Read the model definition and answer for the solid it produces. Units are mm, in the model's axes. Face numbers are marked on the shaded views. A direction names the side the tool comes from. Coordinates: 2 decimals unless noted, no trailing zeros. Loops run counter-clockwise (first coordinate to the right, second up) from the corner with the lowest first, then second, coordinate; pieces in that order, holes last.
from build123d import *

# Parameters (mm, degrees)
SKETCH4_R           = 31.5
SKETCH4_R_2         = 21.5
SKETCH4_R_3         = 2
BOSS_EXTRUDE1_DEPTH = 4
SKETCH5_W           = 97.16267939
SKETCH5_H           = 14.406328081
SKETCH5_H_2         = 19.608613221
CUT_EXTRUDE1_DEPTH  = 66


with BuildPart() as part:
    # Sketch1 → Revolve1 (revolve)
    with BuildSketch(Plane.XY):
        Polygon((-12, 2.5), (-12, -2.5), (-16, -2.5), (-16, -18.5), (-20, -18.5), (-20, -32.5), (-23, -32.5), (-23, 32.5), (-20, 32.5), (-20, 18.5), (-16, 18.5), (-16, 2.5), align=None)
    revolve(axis=Axis((0, 75.096781517, 0), (0, -1, 0)))

    # Sketch4 → Boss-Extrude1 (add)
    with BuildSketch(Plane(origin=(0, 32.5, 0), x_dir=(1, 0, 0), z_dir=(0, 1, 0))):
        Circle(SKETCH4_R)
        Circle(SKETCH4_R_2, mode=Mode.SUBTRACT)
        with Locations((0, 27)):
            Circle(SKETCH4_R_3, mode=Mode.SUBTRACT)
        with Locations((19.091883092, 19.091883092)):
            Circle(SKETCH4_R_3, mode=Mode.SUBTRACT)
        with Locations((27, 0)):
            Circle(SKETCH4_R_3, mode=Mode.SUBTRACT)
        with Locations((19.091883092, -19.091883092)):
            Circle(SKETCH4_R_3, mode=Mode.SUBTRACT)
        with Locations((0, -27)):
            Circle(SKETCH4_R_3, mode=Mode.SUBTRACT)
        with Locations((-19.091883092, -19.091883092)):
            Circle(SKETCH4_R_3, mode=Mode.SUBTRACT)
        with Locations((-27, 0)):
            Circle(SKETCH4_R_3, mode=Mode.SUBTRACT)
        with Locations((-19.091883092, 19.091883092)):
            Circle(SKETCH4_R_3, mode=Mode.SUBTRACT)
    boss_extrude1 = extrude(amount=-BOSS_EXTRUDE1_DEPTH)

    # Mirror1: Boss-Extrude1 across plane
    add(boss_extrude1.mirror(Plane.ZX))

    # Sketch5 → Cut-Extrude1 (cut, through all)
    with BuildSketch(Plane(origin=(0, 32.5, 0), x_dir=(1, 0, 0), z_dir=(0, 1, 0))):
        with Locations((4.630564128, 32.20316404)):
            Rectangle(SKETCH5_W, SKETCH5_H)
        with Locations((4.630564128, -34.804306611)):
            Rectangle(SKETCH5_W, SKETCH5_H_2)
    extrude(amount=-CUT_EXTRUDE1_DEPTH, mode=Mode.SUBTRACT)


solid = part.part
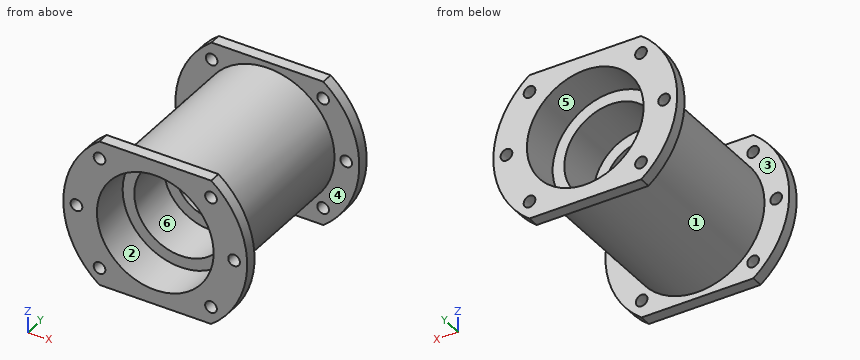
Item 1: Given pin 1 (3 mm diameter, centred on x = 27, z = 0, fed in from +Y); pin 2 (12 mm diameter, centred on x = -5.5, z = -5.5, fed in from -Y); pin 3 (1 mm diameter, centred on y = -24, z = -4.5, fed in from -X); pin 4 (5 mm diameter, centred on x = 17.5, z = 3, fed in from -Y), each flat-ended and moving along its own axis, determine where each tip first touches the part or whether it passes through.
Numbers:
pin 1: passes through
pin 2: stops at y = -2.5
pin 3: stops at x = -22.65
pin 4: stops at y = -32.5
Item 2: A cutting plane is placed at C-C on y = 0.5. Determine the outline of the cut face in (x, z).
Numbers:
outline: circle Ø46 at (0, 0); hole circle Ø24 at (0, 0)
Item 3: Which of the six approach directions +Z, -Z, +X, -X, +Y, -Y give full straight-line access (tool end or side, diameter ignored) to the marked faces 4, 5 and 6?
Numbers:
face 4: none
face 5: +Y
face 6: -Y
Item 4: A cutting plane is placed at B-B on x = -27. Determine the outline of the cut face in (y, z), then the cut area to 3 significant figures.
Numbers:
outline: (-32.5, -16.22) - (-28.5, -16.22) - (-28.5, -2) - (-32.5, -2) - close; (-32.5, 2) - (-28.5, 2) - (-28.5, 16.22) - (-32.5, 16.22) - close; (28.5, -16.22) - (32.5, -16.22) - (32.5, -2) - (28.5, -2) - close; (28.5, 2) - (32.5, 2) - (32.5, 16.22) - (28.5, 16.22) - close
area: 228 mm2
Item 5: A cutting plane is placed at D-D on z = 0. Give the number of separate pieces and of enclosed holes in the cut face, then the cut area to 3 significant figures.
Numbers:
separate pieces: 6
enclosed holes: 0
area: 798 mm2
Item 6: Find the intervals of material crossed by line 1 along Y through (x, z) = (-20.5, -13); line 2 along Z through (x, y) = (0, 8); line 3 along Z through (x, y) = (0, 28), in increasing order.
Numbers:
line 1: y = -32.5 to -28.5, 28.5 to 32.5
line 2: z = -23 to -16, 16 to 23
line 3: z = -23 to -20, 20 to 23
Item 7: Determine the mould class of the marked faces 1, 2 and 3 for opening direction Z: released by +Z, released by -Z, zero draft, split by the parting line, or undercut.
Numbers:
face 1: split by the parting line
face 2: undercut
face 3: zero draft
